Design review of the part built by this model. Coordinates are the model's own, in mm. A direction names the side the tool comes from. Coordinates: 2 decimals unless noted, no trailing zeros. Loops run counter-clockwise (first coordinate to the right, second up) from the corner with the lowest first, then second, coordinate; pieces in that order, holes last. Notation, with made-up numbers: M 15,42 L 48,42 A30 cw 48,69 Z; hole C -18.75,60.5 d7. An arc over 180 degrees is marked long. One line per item, written item: value.
```python
from build123d import *

# Parameters (mm, degrees)
F1_DEPTH = 127
F3_D     = 12.7
F3_DEPTH = 38.1
F5_D     = 12.7
F5_DEPTH = 38.1
F6_W     = 76.2
F6_H     = 19.05
F7_DEPTH = 254.001


with BuildPart() as f1:
    # F0 (on Right) → F1 (new body)
    with BuildSketch(Plane.YZ):
        Polygon((38.1, 0), (0, 0), (0, -63.5), (254, -63.5), (254, -25.4), (38.1, -25.4), align=None)
    extrude(amount=F1_DEPTH)

    # F3
    with Locations(Plane.XZ):
        with Locations((12.7, -12.7)):
            Hole(F3_D / 2, depth=F3_DEPTH)

    # F5
    with Locations(Plane.XZ):
        with Locations((114.3, -12.7)):
            Hole(F5_D / 2, depth=F5_DEPTH)

    # F6 (on face) → F7 (cut, through all)
    with BuildSketch(Plane(origin=(0, 254, 0), x_dir=(-1, 0, 0), z_dir=(0, 1, 0))):
        with Locations((-63.5, -53.975)):
            Rectangle(F6_W, F6_H)
    extrude(amount=-F7_DEPTH, mode=Mode.SUBTRACT)


solid = f1.part
```
(1) We need section D-D on y = 18.5. State the section outline as (x, z) points.
Reply:
outline: M 0,-63.5 L 25.4,-63.5 L 25.4,-44.45 L 101.6,-44.45 L 101.6,-63.5 L 127,-63.5 L 127,0 L 0,0 Z; hole C 12.7,-12.7 d12.7; hole C 114.3,-12.7 d12.7
(2) To check wall thickness, follow line 1 along X through (y, z) = (27, -12); line 2 along Z through (x, y) = (12, 27); line 3 along X through (y, z) = (62.5, -55.5). State the ranges of each line that lie inside material, in increasing order. Write a range as [from, to].
Reply:
line 1: x = [0, 6.39], [19.01, 107.99], [120.61, 127]
line 2: z = [-63.5, -19.01], [-6.39, 0]
line 3: x = [0, 25.4], [101.6, 127]
(3) Tool access review of faces 4 (the flat face through (64, 129, -44.45)), 5 (the flat face through (63, 148, -25.4)), 6 (the flat face through (63, 19, 0)): name each direction out of +Z, -Z, +X, -X, +Y, -Y from which nothing blocks a thin tool from reaching the whole face with its end or side.
Reply:
face 4: -Z, +Y, -Y
face 5: +Z, +X, -X, +Y
face 6: +Z, +X, -X, +Y, -Y
(4) We need section C-C on y = 136. State the section outline as (x, z) points.
Reply:
outline: M 0,-63.5 L 25.4,-63.5 L 25.4,-44.45 L 101.6,-44.45 L 101.6,-63.5 L 127,-63.5 L 127,-25.4 L 0,-25.4 Z
(5) Insertion check: pin 1 (10 mm diameter, centred on x = 62.5, y = 224, fed in from -Z); pin 2 (1 mm diameter, centred on x = 102, z = -18.5, fed in from +Y). Each pin has a flat end and moves straight along its axis. Give the tip position at first contact, or say it passes through.
Reply:
pin 1: stops at z = -44.45
pin 2: stops at y = 38.1
(6) Mouldability with a two-part tool opening along X and no side actions: class faces 1 (the flat face through (63, 38.1, -13)), 2 (the flat face through (101.6, 129, -54)), 3 (the flat face through (127, 125, -45)) as released by +X, released by -X, zero draft, split by the parting line, or undercut.
Reply:
face 1: zero draft
face 2: undercut
face 3: released by +X
(7) We need section B-B on x = 12.7. State the section outline as (y, z) points.
Reply:
outline: M 0,-63.5 L 254,-63.5 L 254,-25.4 L 38.1,-25.4 L 38.1,-19.05 L 0,-19.05 Z; M 0,-6.35 L 38.1,-6.35 L 38.1,0 L 0,0 Z
(8) We need section A-A on z = -12.7. State the section outline as (x, y) points.
Reply:
outline: M 0,0 L 6.35,0 L 6.35,38.1 L 0,38.1 Z; M 19.05,0 L 107.95,0 L 107.95,38.1 L 19.05,38.1 Z; M 120.65,0 L 127,0 L 127,38.1 L 120.65,38.1 Z
